Autodesk Inventor part; units mm, degrees
ref_plane "YZ Plane" through (0, 0, 0) normal (1, 0, 0) x (0, 1, 0)
ref_plane "XZ Plane" through (0, 0, 0) normal (0, 1, 0) x (-1, 0, 0)
ref_plane "XY Plane" through (0, 0, 0) normal (0, 0, 1) x (1, 0, 0)
sketch "Esquisse2" plane through (0, 0, 0) normal (0, 0, 1) x (1, 0, 0)
  circle A0 centre (0, 0) radius 100
  dimension "Diamètre" = 200
extrude "Embase" add sketch "Esquisse2" against normal blind 3
sketch "Esquisse1" plane through (0, 0, 0) normal (0, 0, 1) x (1, 0, 0)
  arc A0 (99.7184, -7.5) -> (95.3938, 30.0004) centre (0, 0) ccw
  arc A1 (119.4999, -0.1943) -> (95.3938, 30.0004) centre (89.51, 0.583) ccw
  line L0 (99.7184, -7.5) -> (112.0024, -7.5)
  arc A2 (112.0024, -7.5) -> (119.4999, -0.1943) centre (112.0024, 0) ccw
  point P0 (106.4504, 15)
  point P1 (106.4504, 15)
  dimension "d0" = 200
  dimension "d1" = 60
  dimension "d2" = 89.51
  dimension "d3" = 0.583
  dimension "d4" = 7.5
  dimension "d5" = 15
  dimension "d9" = 15
  dimension "d10" = 5.552
extrude "Oreille" add sketch "Esquisse1" against normal up to surface (3 mm away)
hole "M3" at (106.4504, 15, 0) direction (0, 0, -1) diameter 2.459 depth 8.8 tip angle 118
hole "Passage vis" at (112.0024, 0, 0) direction (0, 0, -1) diameter 5.5 end through all
fillet "Congé1" radius 8 2 edges at (99.7184, -7.5, -1.5) (95.3938, 30.0004, -1.5)
pattern_circular "Réseau circulaire1" count 3 over 360 about axis through (0, 0, -10) along (0, 0, 1) of "Congé1", "Passage vis", "M3", "Oreille"
equation "\"d0\" = Diamètre"
properties part number "Plateau metalique" material "Aluminium"
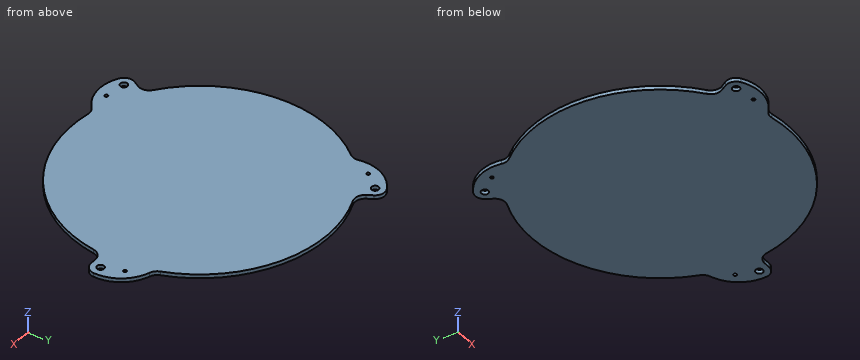
Geometry check sheet. Reference: the model listing, model coordinates, mm. Round coordinates to 2 decimals unless told otherwise and drop trailing zeros. Loops run counter-clockwise (first coordinate to the right, second up) from the corner with the lowest first, then second, coordinate; pieces in that order, holes last. Notation, with made-up numbers: (13.5, 80.5) - (21.5, 80.5) arc R27 cw to (21.5, 112.5) - close; hole circle Ø6 at (31.5, 69). An arc over 180 degrees is marked (long way). Use a Markdown table: item, result.
Q1. Cross-section at A-A on x = -71. Record the cut outline in (y, z), plus the area to 3 significant figures.
Solutions:
| item | result |
|---|---|
| outline | (-70.42, -3) - (92.64, -3) - (92.64, 0) - (-70.42, 0) - close |
| area | 489 mm2 |
Q2. Cross-section at C-C on y = -40. Record the cut outline in (x, z), plus the area to 3 significant figures.
Solutions:
| item | result |
|---|---|
| outline | (-91.65, -3) - (91.65, -3) - (91.65, 0) - (-91.65, 0) - close |
| area | 550 mm2 |
Q3. Material ranges on line 1 (X direction, y = 0, z = -0.8); line 2 (X direction, y = 1.5, z = -2.55); line 3 (Y direction, x = -40, z = -1.95), recorded low to high.
Solutions:
| item | result |
|---|---|
| line 1 | x = -100 to 109.25, 114.75 to 119.5 |
| line 2 | x = -99.99 to 109.7, 114.31 to 119.5 |
| line 3 | y = -107.51 to -100.9, -98.48 to 92.31 |
Q4. Cross-section at B-B on z = -2.5. State how many separate pieces and enclosed holes the cut face has, plus the area to 3 significant figures.
Solutions:
| item | result |
|---|---|
| separate pieces | 1 |
| enclosed holes | 6 |
| area | 33,100 mm2 |
Q5. Go/stop test with a flat-tipped pin: P1, Ø1.5, axis at x = 108.5, z = -1.5, coming from the -Y side. Record where the tip stops, or that it passes through.
Solutions:
| item | result |
|---|---|
| P1 | stops at y = -7.5 |
